Autodesk Inventor part; units mm, degrees
ref_plane "YZ Plane" through (0, 0, 0) normal (1, 0, 0) x (0, 1, 0)
ref_plane "XZ Plane" through (0, 0, 0) normal (0, 1, 0) x (-1, 0, 0)
ref_plane "XY Plane" through (0, 0, 0) normal (0, 0, 1) x (1, 0, 0)
sketch "Sketch1" plane through (0, 0, 0) normal (1, 0, 0) x (0, 1, 0)
  line L0 (4.25, 20) -> (30.75, 20)
  line L1 (30.75, 20) -> (30.75, 12)
  line L2 (30.75, 12) -> (35, 12)
  line L3 (35, 12) -> (35, 0)
  line L4 (35, 0) -> (16.25, 0)
  line L5 (16.25, 0) -> (16.25, -5)
  line L6 (16.25, -5) -> (8.75, -5)
  line L7 (8.75, -5) -> (8.75, 0)
  line L8 (8.75, 0) -> (0, 0)
  line L9 (0, 0) -> (0, 12)
  line L10 (0, 12) -> (4.25, 12)
  line L11 (4.25, 12) -> (4.25, 20)
  line L12 (3.5429, 12) -> (4.25, 12.7071)
  line L13 (4.25, 12.7071) -> (4.9571, 12)
  line L14 (4.9571, 12) -> (4.25, 11.2929)
  line L15 (4.25, 11.2929) -> (3.5429, 12)
  line L16 (30.75, 12.7071) -> (31.4571, 12)
  line L17 (31.4571, 12) -> (30.75, 11.2929)
  line L18 (30.75, 11.2929) -> (30.0429, 12)
  line L19 (30.0429, 12) -> (30.75, 12.7071)
  dimension "d0" = 35
  dimension "d3" = 7.5
  dimension "d4" = 8
  dimension "d5" = 25
  dimension "d6" = 5
  dimension "d7" = 22
  dimension "d9" = 12
  dimension "d11" = 4.25
  dimension "d12" = 4.25
  dimension "d19" = 1
  dimension "d20" = 0.5
  dimension "d21" = 0.5
  dimension "d22" = 1
  dimension "d23" = 45
extrude "Extrusion1" add sketch "Sketch1" along normal mid plane 50 contours L0 L1 L19 L18 L17 L2 L3 L4 L5 L6 L7 L8 L9 L10 L15 L14 L13 L11
sketch "Sketch2" plane through (-25, 0, 0) normal (0, -1, 0) x (1, 0, 0)
  line L0 (0, 20) -> (12.5, 20)
  line L1 (12.5, 20) -> (12.5, 12)
  line L2 (12.5, 12) -> (0, 12)
  line L3 (0, 12) -> (0, 20)
  line L4 (37.5, 20) -> (50, 20)
  line L5 (50, 20) -> (50, 12)
  line L6 (50, 12) -> (37.5, 12)
  line L7 (37.5, 12) -> (37.5, 20)
  line L8 (50, -5) -> (35, -5)
  line L9 (35, -5) -> (35, 0)
  line L10 (35, 0) -> (50, 0)
  line L11 (50, 0) -> (50, -5)
  line L12 (0, -5) -> (15, -5)
  line L13 (15, -5) -> (15, 0)
  line L14 (15, 0) -> (0, 0)
  line L15 (0, 0) -> (0, -5)
  line L16 (0, -5) -> (50, -5)
  line L17 (50, 0) -> (50, -5)
  line L18 (50, 20) -> (0, 20)
  line L19 (0, 12.7071) -> (0, 20)
  line L20 (0, 12) -> (50, 12)
  line L21 (25, 0) -> (50, 0)
  dimension "d15" = 25
  dimension "d16" = 20
extrude "Extrusion2" cut sketch "Sketch2" against normal through all contours L0 L1 L2 L3 | L4 L5 L6 L7 | L12 L15 L14 L13 | L8 L9 L10 L11
sketch "Sketch4" plane through (12.5, 30.0429, 12) normal (0, 0, 1) x (1, 0, 0)
  line L0 (-31.5, -19.0429) -> (-31.5, -16.0429) construction
  line L1 (-28.25, -19.0429) -> (-28.25, -16.0429)
  line L2 (-34.75, -16.0429) -> (-34.75, -19.0429)
  arc A0 (-34.75, -19.0429) -> (-28.25, -19.0429) centre (-31.5, -19.0429) ccw
  arc A1 (-28.25, -16.0429) -> (-34.75, -16.0429) centre (-31.5, -16.0429) ccw
  line L3 (-37.5, -25.0858) -> (-37.5, 0)
  line L4 (-22.5, -21.2929) -> (-2.5, -21.2929)
  point P0 (-31.5, -17.5429)
  dimension "d24" = 6.5
  dimension "d25" = 3
  dimension "d26" = 6
  dimension "d27" = 3.75
extrude "Extrusion3" cut sketch "Sketch4" against normal through all
mirror "Mirror1" about plane through (0, 0, 0) normal (1, 0, 0) of "Extrusion3"
equation "\"d21\" = d20"
equation "\"d22\" = d19"
properties part number "Holding Block" material "Aluminum 6061"
Build history of the part. All positions in model axes, mm. A direction names the side the tool comes from. Round coordinates to 2 decimals unless told otherwise and drop trailing zeros. Write each loop counter-clockwise with the first axis right and the second up, starting at its lowest first coordinate (ties: lowest second). Pieces come first, ordered by that corner, then holes. Notation, with made-up numbers: M -5.75,-31.75 L 7.25,-31.75 A33 cw 7.25,7.25 Z; hole C 81.5,13.5 d7. An arc over 180 degrees is marked long. Answer as a JSON object with one key per item and string values. Group by question number.
(1) Mould opens along X. For faces 4 (the flat face through (12.5, 17, 16)), 5 (the flat face through (-25, 17, 6)), 6 (the flat face through (22.25, 12, 6)) say: pulls with the +X half, pulls with the -X half, needs draft (parallel to the pull), parting line crosses it, or undercut.
(2) Drill centre lines: L1, parallel to Y at x = 8, z = 11.5; L2, parallel to Y at x = 4, z = -3.5; L3, parallel to Z at x = -22.5, y = 26. Where is each one in solid material? Low to high.
(3) Flat gauge pins, fed straight in: pin 1 (14 mm diameter, centred on x = 21, y = 22, fed in from +Z); pin 2 (4 mm diameter, centred on x = -16, y = 18, fed in from -Z); pin 3 (2.5 mm diameter, centred on y = 12.5, z = -3.5, fed in from +X). Where does each tip first touch, or does it go through?
(4) Cut at A-A (x = -19). Give the cut face in (y, z), and give its area (3 significant figures).
(5) Cut at D-D (y = 20). Give the cut face in (x, z).
(6) Which spindle directions (+Z, -Z, +X, -X, +Y, -Y) get a long thin tool onto all of the face, cutting with end or side? Do faces 1 (the flat face through (-22.25, 13, 6)), 2 (the flat face through (10, 12, -3)), 3 (the flat face through (-10, 12, -3)). Say none if no direction does.
(7) Cut at B-B (z = 4). Give the cut face in (x, y).
(8) Cut at C-C (y = 15.5). Give the cut face in (x, z).
Responses:
{
 "1": {"face 4": "pulls with the +X half", "face 5": "pulls with the -X half", "face 6": "undercut"},
 "2": {"L1": "y = 0 to 4.04, 4.46 to 30.54, 30.96 to 35", "L2": "y = 8.75 to 16.25", "L3": "z = 0 to 12"},
 "3": {"pin 1": "stops at z = 12", "pin 2": "stops at z = 0", "pin 3": "stops at x = 10"},
 "4": {"outline": "M 0,0 L 7.75,0 L 7.75,12 L 4.96,12 L 4.25,11.29 L 3.54,12 L 0,12 Z; M 17.25,0 L 35,0 L 35,12 L 31.46,12 L 30.75,11.29 L 30.04,12 L 17.25,12 Z", "area": "305 mm2"},
 "5": {"outline": "M -25,0 L 25,0 L 25,12 L 12.5,12 L 12.5,20 L -12.5,20 L -12.5,12 L -25,12 Z"},
 "6": {"face 1": "+Z, -Z", "face 2": "-Z, +X, +Y, -Y", "face 3": "-Z, -X, +Y, -Y"},
 "7": {"outline": "M -25,0 L 25,0 L 25,35 L -25,35 Z; hole M -22.25,11 A3.25 ccw -15.75,11 L -15.75,14 A3.25 ccw -22.25,14 Z; hole M 15.75,11 A3.25 ccw 22.25,11 L 22.25,14 A3.25 ccw 15.75,14 Z"},
 "8": {"outline": "M -25,0 L -21.88,0 L -21.88,12 L -25,12 Z; M -16.12,0 L -10,0 L -10,-5 L 10,-5 L 10,0 L 16.12,0 L 16.12,12 L 12.5,12 L 12.5,20 L -12.5,20 L -12.5,12 L -16.12,12 Z; M 21.88,0 L 25,0 L 25,12 L 21.88,12 Z"}
}
